Read the model definition and answer for the solid it produces. Units are mm, in the model's axes. Round coordinates to 2 decimals unless told otherwise and drop trailing zeros. Write each loop counter-clockwise with the first axis right and the second up, starting at its lowest first coordinate (ties: lowest second). Pieces come first, ordered by that corner, then holes. Notation, with made-up numbers: (26, -12.75) - (37, -12.75) arc R7 ccw to (37, -0.75) - close; hole circle Ø7 at (70, -20.5). An arc over 180 degrees is marked (long way). One line per item, written item: value. Start each with the question number.
(1) Find the intervals of material crossed by L1, parallel to Y at x = 0, z = 4; L2, parallel to Y at x = 0.8, z = 1.25; L3, parallel to X at y = 0.35, z = 3, in increasing order.
(2) A cutting plane is placed at C-C, the plane z = 9.25. Determine the outline of the cut face in (x, y).
(3) A cutting plane is placed at A-A, the plane x = 0. Determine the outline of the cut face in (y, z).
(4) The mould has two halves that part along Y. Classify faces 1 (the face through (0, -3, 6)), 2 (the face through (-1.43, -0.45, 5.67)), 3 (the face through (0, 3, 6)), 4 (the face through (-3, 0, 6)): +Y half, -Y half, draft (parallel to the pull), parting line (faces both ways), or undercut.
from build123d import *

# Parameters (mm, degrees)
ESQUISSE1_R      = 1.5
EXTRUSION1_DEPTH = 11.5
CONG_1_R         = 0.2


with BuildPart() as part:
    # Esquisse1 → Extrusion1 (new body)
    with BuildSketch(Plane.XY):
        with BuildLine():
            Line((-2.8, 3), (2.8, 3))
            ThreePointArc((2.8, 3), (2.941421356, 2.941421356), (3, 2.8))
            Line((3, 2.8), (3, -2.8))
            ThreePointArc((3, -2.8), (2.941421356, -2.941421356), (2.8, -3))
            Line((2.8, -3), (-2.8, -3))
            ThreePointArc((-2.8, -3), (-2.941421356, -2.941421356), (-3, -2.8))
            Line((-3, -2.8), (-3, 2.8))
            ThreePointArc((-3, 2.8), (-2.941421356, 2.941421356), (-2.8, 3))
        make_face()
        with Locations(Location((0, 0, 0), (0, 0, 180))):
            Circle(ESQUISSE1_R, mode=Mode.SUBTRACT)
    extrude(amount=EXTRUSION1_DEPTH)

    # Congé1
    cong_1_edges = [part.edges().sort_by_distance(p)[0] for p in [
        (0, 3, 0),
        (0, 3, 11.5),
        (2.941421356, 2.941421356, 0),
        (2.941421356, 2.941421356, 11.5),
        (3, 0, 0),
        (3, 0, 11.5),
        (2.941421356, -2.941421356, 0),
        (2.941421356, -2.941421356, 11.5),
        (0, -3, 0),
        (0, -3, 11.5),
        (-2.941421356, -2.941421356, 0),
        (-2.941421356, -2.941421356, 11.5),
        (-3, 0, 0),
        (-3, 0, 11.5),
        (-2.941421356, 2.941421356, 0),
        (-2.941421356, 2.941421356, 11.5),
        (1.5, 0, 0),
        (1.5, 0, 11.5),
    ]]
    fillet(cong_1_edges, radius=CONG_1_R)


solid = part.part
Here are the results:
1. L1: -3 to -1.5, 1.5 to 3
1. L2: -3 to -1.27, 1.27 to 3
1. L3: -3 to -1.46, 1.46 to 3
2. outline: (-3, -2.8) arc R0.2 ccw to (-2.8, -3) - (2.8, -3) arc R0.2 ccw to (3, -2.8) - (3, 2.8) arc R0.2 ccw to (2.8, 3) - (-2.8, 3) arc R0.2 ccw to (-3, 2.8) - close; hole circle Ø3 at (0, 0)
3. outline: (-3, 0.2) arc R0.2 ccw to (-2.8, 0) - (-1.7, 0) arc R0.2 ccw to (-1.5, 0.2) - (-1.5, 11.3) arc R0.2 ccw to (-1.7, 11.5) - (-2.8, 11.5) arc R0.2 ccw to (-3, 11.3) - close; (1.5, 0.2) arc R0.2 ccw to (1.7, 0) - (2.8, 0) arc R0.2 ccw to (3, 0.2) - (3, 11.3) arc R0.2 ccw to (2.8, 11.5) - (1.7, 11.5) arc R0.2 ccw to (1.5, 11.3) - close
4. face 1: -Y half
4. face 2: undercut
4. face 3: +Y half
4. face 4: draft
